from build123d import *

# Parameters (mm, degrees)
BOX_W            = 101.6
BOX_H            = 48.26
BOX_DEPTH        = 19.05
FILLET_R         = 0.254
HOLE_D           = 3.9
HOLE_DEPTH       = 13.446125
HOLE_CSINK_D     = 5.1816
HOLE_CSINK_ANGLE = 82
HOLE_TIPS_R      = 1.95
POCKET_DEPTH     = 12.7
FILLET001_R      = 0.254


with BuildPart() as part:
    # Box → Box (join)
    with BuildSketch(Plane.XY):
        with Locations((50.8, 24.13)):
            Rectangle(BOX_W, BOX_H)
    extrude(amount=BOX_DEPTH)

    # Fillet
    fillet_edges = [part.edges().sort_by_distance(p)[0] for p in [
        (0, 0, 9.525),
        (0, 48.26, 9.525),
        (101.6, 48.26, 9.525),
        (101.6, 0, 9.525),
    ]]
    fillet(fillet_edges, radius=FILLET_R)

    # Hole
    with Locations(Plane.XY.offset(19.05)):
        with Locations((3.81, 44.45), (97.79, 44.45), (29.21, 40.64), (72.39, 40.64), (3.81, 3.81), (97.79, 3.81), (50.8, 17.3736)):
            CounterSinkHole(HOLE_D / 2, HOLE_CSINK_D / 2, depth=HOLE_DEPTH, counter_sink_angle=HOLE_CSINK_ANGLE)

    # Hole tips → Hole tip 1 section 0
    with BuildSketch(Plane.XY.offset(5.603875), mode=Mode.PRIVATE) as hole_tip_1_s0:
        with Locations((3.81, 44.45)):
            Circle(HOLE_TIPS_R)
    loft([hole_tip_1_s0.sketch, Vertex(3.81, 44.45, 4.432197)], mode=Mode.SUBTRACT)

    # Hole tips → Hole tip 2 section 0
    with BuildSketch(Plane.XY.offset(5.603875), mode=Mode.PRIVATE) as hole_tip_2_s0:
        with Locations((97.79, 44.45)):
            Circle(HOLE_TIPS_R)
    loft([hole_tip_2_s0.sketch, Vertex(97.79, 44.45, 4.432197)], mode=Mode.SUBTRACT)

    # Hole tips → Hole tip 3 section 0
    with BuildSketch(Plane.XY.offset(5.603875), mode=Mode.PRIVATE) as hole_tip_3_s0:
        with Locations((29.21, 40.64)):
            Circle(HOLE_TIPS_R)
    loft([hole_tip_3_s0.sketch, Vertex(29.21, 40.64, 4.432197)], mode=Mode.SUBTRACT)

    # Hole tips → Hole tip 4 section 0
    with BuildSketch(Plane.XY.offset(5.603875), mode=Mode.PRIVATE) as hole_tip_4_s0:
        with Locations((72.39, 40.64)):
            Circle(HOLE_TIPS_R)
    loft([hole_tip_4_s0.sketch, Vertex(72.39, 40.64, 4.432197)], mode=Mode.SUBTRACT)

    # Hole tips → Hole tip 5 section 0
    with BuildSketch(Plane.XY.offset(5.603875), mode=Mode.PRIVATE) as hole_tip_5_s0:
        with Locations((3.81, 3.81)):
            Circle(HOLE_TIPS_R)
    loft([hole_tip_5_s0.sketch, Vertex(3.81, 3.81, 4.432197)], mode=Mode.SUBTRACT)

    # Hole tips → Hole tip 6 section 0
    with BuildSketch(Plane.XY.offset(5.603875), mode=Mode.PRIVATE) as hole_tip_6_s0:
        with Locations((97.79, 3.81)):
            Circle(HOLE_TIPS_R)
    loft([hole_tip_6_s0.sketch, Vertex(97.79, 3.81, 4.432197)], mode=Mode.SUBTRACT)

    # Hole tips → Hole tip 7 section 0
    with BuildSketch(Plane.XY.offset(5.603875), mode=Mode.PRIVATE) as hole_tip_7_s0:
        with Locations((50.8, 17.3736)):
            Circle(HOLE_TIPS_R)
    loft([hole_tip_7_s0.sketch, Vertex(50.8, 17.3736, 4.432197)], mode=Mode.SUBTRACT)

    # Sketch (on Face2 of Hole) → Pocket (cut)
    with BuildSketch(Plane.XY.offset(19.05)):
        with BuildLine():
            Line((7.62, 12.573), (7.62, 35.687))
            ThreePointArc((12.573, 40.64), (9.0707, 39.1893), (7.62, 35.687))
            Line((12.573, 40.64), (17.295288, 40.64))
            ThreePointArc((21.868849, 37.58825), (20.044408, 39.807018), (17.295288, 40.64))
            ThreePointArc((21.868849, 37.58825), (29.21, 32.6898), (36.551151, 37.58825))
            ThreePointArc((41.124712, 40.64), (38.375592, 39.807018), (36.551151, 37.58825))
            Line((41.124712, 40.64), (60.475288, 40.64))
            ThreePointArc((65.048849, 37.58825), (63.224408, 39.807018), (60.475288, 40.64))
            ThreePointArc((65.048849, 37.58825), (72.39, 32.6898), (79.731151, 37.58825))
            ThreePointArc((84.304712, 40.64), (81.555592, 39.807018), (79.731151, 37.58825))
            Line((84.304712, 40.64), (89.027, 40.64))
            ThreePointArc((93.98, 35.687), (92.5293, 39.1893), (89.027, 40.64))
            Line((93.98, 35.687), (93.98, 12.573))
            ThreePointArc((89.027, 7.62), (92.5293, 9.0707), (93.98, 12.573))
            Line((89.027, 7.62), (69.358352, 7.62))
            ThreePointArc((65.856052, 9.0707), (67.462921, 7.997025), (69.358352, 7.62))
            Line((65.856052, 9.0707), (54.176576, 20.750176))
            ThreePointArc((54.176576, 20.750176), (50.8, 22.1488), (47.423424, 20.750176))
            Line((47.423424, 20.750176), (35.743948, 9.0707))
            ThreePointArc((32.241648, 7.62), (34.137079, 7.997025), (35.743948, 9.0707))
            Line((32.241648, 7.62), (12.573, 7.62))
            ThreePointArc((7.62, 12.573), (9.0707, 9.0707), (12.573, 7.62))
        make_face()
        with BuildLine():
            Line((38.8961, 1.4507), (47.2977, 9.8523))
            ThreePointArc((54.3023, 9.8523), (50.8, 11.303), (47.2977, 9.8523))
            Line((54.3023, 9.8523), (62.7039, 1.4507))
            ThreePointArc((62.7039, 1.4507), (64.310769, 0.377025), (66.2062, 0))
            Line((35.3938, 0), (66.2062, 0))
            ThreePointArc((35.3938, 0), (37.289231, 0.377025), (38.8961, 1.4507))
        make_face()
    extrude(amount=-POCKET_DEPTH, mode=Mode.SUBTRACT)

    # Fillet001
    fillet001_edges = [part.edges().sort_by_distance(p)[0] for p in [
        (17.8239, 0, 19.05),
        (22.407324, 7.62, 19.05),
    ]]
    fillet(fillet001_edges, radius=FILLET001_R)


solid = part.part
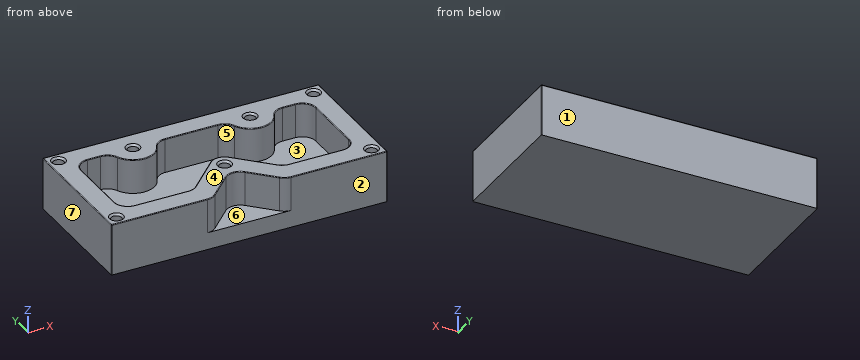
The model under review builds one solid part; all positions refer to its coordinate system, in mm. Face numbers are marked on the shaded views. A direction names the side the tool comes from. Give positions to 0.01 mm unless a question says otherwise; leave off trailing zeros. Write each loop counter-clockwise with the first axis right and the second up, starting at its lowest first coordinate (ties: lowest second). Pieces come first, ordered by that corner, then holes.
1. Add section A-A, the plane y = 23.5. Write out the cut boundary in (x, z), plus the area to 3 significant figures.
2. Wall thickness on L1, parallel to Y at x = 3.81, z = 8; L2, parallel to X at y = 44.45, z = 11.5; L3, parallel to Y at x = 50.8, z = 15.75: over which ranges is each line inside the solid? List them lowest first.
3. Draft analysis for pull direction Y (two halves, no side actions). For the marked faces 1, 2, 3 and 4, state which applies: +Y half, -Y half, draft (parallel to the pull), parting line (faces both ways), or undercut.
4. For P1, Ø6, axis at x = 46.5, z = 14, coming from the -Y side; P2, Ø5, axis at x = 20, y = 35, coming from the +Z side; P3, Ø4.5, axis at x = 3.81, y = 3.81, coming from the +Z side, all flat-tipped, find the tip position at first contact; note any pin that passes through.
5. Tool access review of the marked faces 5, 6 and 7: name each direction out of +Z, -Z, +X, -X, +Y, -Y from which nothing blocks a thin tool from reaching the whole face with its end or side.
6. Add section B-B, the plane z = 12.5. Count the separate pieces of the cut face and the enclosed holes in it, plus the area to 3 significant figures.
Worked answers:
1. outline: (0, 0) - (101.6, 0) - (101.6, 18.8) arc R0.25 ccw to (101.35, 19.05) - (94.23, 19.05) arc R0.25 ccw to (93.98, 18.8) - (93.98, 6.35) - (7.62, 6.35) - (7.62, 18.8) arc R0.25 ccw to (7.37, 19.05) - (0.25, 19.05) arc R0.25 ccw to (0, 18.8) - close
1. area: 839 mm2
2. L1: y = 0 to 1.86, 5.76 to 42.5, 46.4 to 48.26
2. L2: x = 0 to 1.86, 5.76 to 95.84, 99.74 to 101.6
2. L3: y = 11.3 to 15.42, 19.32 to 22.15, 40.64 to 48.26
3. face 1: +Y half
3. face 2: -Y half
3. face 3: undercut
3. face 4: draft
4. P1: stops at y = 6.05
4. P2: stops at z = 6.35
4. P3: stops at z = 18.66
5. face 5: +Z
5. face 6: +Z, -Y
5. face 7: +Z, -Z, -X, +Y, -Y
6. separate pieces: 1
6. enclosed holes: 8
6. area: 2,290 mm2
